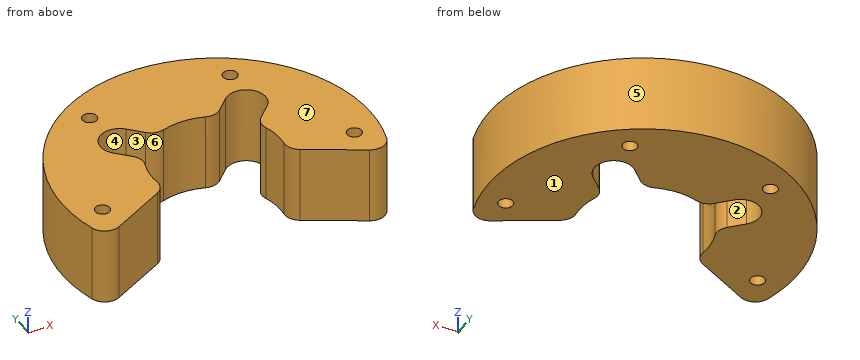
Autodesk Inventor part; units mm, degrees
ref_plane "YZ Plane" through (0, 0, 0) normal (1, 0, 0) x (0, 1, 0)
ref_plane "XZ Plane" through (0, 0, 0) normal (0, 1, 0) x (-1, 0, 0)
ref_plane "XY Plane" through (0, 0, 0) normal (0, 0, 1) x (1, 0, 0)
sketch "Sketch1" plane through (0, 0, 0) normal (0, 0, 1) x (1, 0, 0)
  circle A0 centre (0, 0) radius 60
  circle A1 centre (0, -84) radius 72 construction
  circle A2 centre (0, 0) radius 12 construction
  line L0 (0, -84) -> (0, 0) construction
  line L1 (0, 0) -> (0, 60) construction
  circle A3 centre (0, 0) radius 35 construction
  circle A4 centre (0, 0) radius 50 construction
  line L2 (-50.3895, -32.5714) -> (-8.3983, 8.5714) construction
  line L3 (8.3983, 8.5714) -> (50.3895, -32.5714) construction
  circle A5 centre (0, 0) radius 25
  circle A6 centre (0, 0) radius 60
  line L4 (-50.3895, -32.5714) -> (-24.0638, -6.7776)
  line L5 (24.0638, -6.7776) -> (50.3895, -32.5714)
  circle A7 centre (-24.7487, 24.7487) radius 7.5
  circle A8 centre (24.7487, 24.7487) radius 7.5
  line L6 (-24.7487, 24.7487) -> (24.7487, 24.7487) construction
  circle A9 centre (-24.7487, -24.7487) radius 7.5 construction
  circle A10 centre (24.7487, -24.7487) radius 7.5 construction
  line L7 (-24.7487, 24.7487) -> (-24.7487, -24.7487) construction
  line L8 (24.7487, -24.7487) -> (24.7487, 24.7487) construction
  line L9 (24.7487, -24.7487) -> (-24.7487, -24.7487) construction
  line L10 (-30.052, 19.4454) -> (-22.1667, 11.5601)
  line L11 (-19.4454, 30.052) -> (-11.5601, 22.1667)
  line L12 (19.4454, 30.052) -> (11.5601, 22.1667)
  line L13 (30.052, 19.4454) -> (22.1667, 11.5601)
  line L14 (-49.2404, -8.6824) -> (0, 0) construction
  line L15 (-55.0993, -23.75) -> (-24.0638, -6.7776)
  line L16 (24.0638, -6.7776) -> (55.0993, -23.75)
  point P0 (-27.4754, 41.7744)
  point P1 (27.4754, 41.7744)
  point P2 (49.2404, -8.6824)
  dimension "d0" = 120
  dimension "d4" = 100
  dimension "d1" = 144
  dimension "d2" = 24
  dimension "d3" = 70
  dimension "d5" = 50
  dimension "d6" = 15
  dimension "d7" = 15
  dimension "d8" = 15
  dimension "d9" = 15
  dimension "d10" = 45
  dimension "d11" = 45
  dimension "d12" = 100
  dimension "d15" = 200
  dimension "d30" = 10
  dimension "d32" = 10
extrude "Extrusion1" add sketch "Sketch1" along normal blind 30 contours A0 L16 A5 L13 A8 L12 L11 A7 L10 L15
fillet "Fillet1" radius 6 8 edges at (24.0638, -6.7776, 15) (-24.0638, -6.7776, 15) (-22.1667, 11.5601, 15) (-11.5601, 22.1667, 15) (11.5601, 22.1667, 15) (22.1667, 11.5601, 15) (-55.0993, -23.75, 15) (55.0993, -23.75, 15)
hole "Hole1" at (-49.2404, -8.6824, 0) at (-27.4754, 41.7744, 0) at (27.4754, 41.7744, 0) at (49.2404, -8.6824, 0) direction (0, 0, 1) diameter 5.6 end through all
properties part number "RT_ARM_MC_008_Capstand_Support"
CAD build for the part. Positions are in the model's coordinates, mm. Face numbers are marked on the shaded views. A direction names the side the tool comes from. Round coordinates to 2 decimals unless told otherwise and drop trailing zeros. Loops run counter-clockwise (first coordinate to the right, second up) from the corner with the lowest first, then second, coordinate; pieces in that order, holes last. Notation, with made-up numbers: M 83,57 L 127,57 A16 ccw 127,71 Z; hole C 59.5,4.25 d10. An arc over 180 degrees is marked long. Return JSON: item names as keys, results as strings. Group by question number.
(1) Saw through at B-B, the plane z = 9.75. List the corners of the cut face in (x, y), and give its area (3 significant figures).
(2) Wall check: probe 1 along X at (y, z) = (-10.5, 23.5); probe 2 along X at (y, z) = (30.5, 18.5); probe 3 along Y at (x, z) = (28, 28.5). Give the ranges that are in metal, low to high. Write a range as [from, to].
(3) Drop flat-ended pins along their axis: P1, Ø10, axis at y = 31, z = 10, coming from the +X side; P2, Ø10, axis at y = 5, z = 16.5, coming from the +X side; P3, Ø10, axis at y = 48, z = 14, coming from the +X side. Give the stop position or say it passes through.
(4) Mould opens along Y. For the marked faces 4, 5, 6 and 7 say: +Y half, -Y half, draft (parallel to the pull), parting line (faces both ways), or undercut.
(5) Saw through at C-C, the plane x = 0. List the corners of the cut face in (y, z).
(6) Saw through at A-A, the plane y = 0. List the corners of the cut face in (x, z).
(7) Tool access for the marked faces 1, 2 and 3: list every direction of +Z, -Z, +X, -X, +Y, -Y with a clear straight run to the whole face (end or side of a thin tool).
(8) Saw through at D-D, the plane y = 27. List the corners of the cut face in (x, z).
Answer list:
{
 "1": {"outline": "M -57.6,-16.81 A6 ccw -48.96,-20.39 L -27.91,-8.88 A6 ccw -24.83,-2.92 A25 cw -23.61,8.22 A6 ccw -25.04,14.43 L -30.05,19.45 A7.5 cw -19.45,30.05 L -14.43,25.04 A6 ccw -8.22,23.61 A25 cw 8.22,23.61 A6 ccw 14.43,25.04 L 19.45,30.05 A7.5 cw 30.05,19.45 L 25.04,14.43 A6 ccw 23.61,8.22 A25 cw 24.83,-2.92 A6 ccw 27.91,-8.88 L 48.96,-20.39 A6 ccw 57.6,-16.81 A60 ccw long Z; hole C -49.24,-8.68 d5.6; hole C -27.48,41.77 d5.6; hole C 27.48,41.77 d5.6; hole C 49.24,-8.68 d5.6", "area": "5,140 mm2"},
 "2": {"probe 1": "[-59.07, -51.37], [-47.11, -30.87], [30.87, 47.11], [51.37, 59.07]", "probe 2": "[-51.67, -29.56], [-19.93, 19.93], [29.56, 51.67]", "probe 3": "[-8.93, 17.39], [31.51, 39.02], [44.52, 53.07]"},
 "3": {"P1": "x = 54.07", "P2": "x = 60", "P3": "x = 41.84"},
 "4": {"face 4": "undercut", "face 5": "parting line", "face 6": "-Y half", "face 7": "draft"},
 "5": {"outline": "M 25,0 L 60,0 L 60,30 L 25,30 Z"},
 "6": {"outline": "M -60,0 L -25,0 L -25,30 L -60,30 Z; M 25,0 L 60,0 L 60,30 L 25,30 Z"},
 "7": {"face 1": "-Z, +X, -X, +Y, -Y", "face 2": "+Z, -Z", "face 3": "+Z, -Z, -Y"},
 "8": {"outline": "M -53.58,0 L -31.9,0 L -31.9,30 L -53.58,30 Z; M -16.39,0 L 16.39,0 L 16.39,30 L -16.39,30 Z; M 31.9,0 L 53.58,0 L 53.58,30 L 31.9,30 Z"}
}
